from build123d import *

# Parameters (mm, degrees)
SKETCH1_R           = 2.5
SKETCH1_R_2         = 2
BOSS_EXTRUDE1_DEPTH = 0.5
SKETCH3_R           = 2.25
SKETCH3_R_2         = 1.25
BOSS_EXTRUDE2_DEPTH = 6.2
SKETCH5_R           = 3
BOSS_EXTRUDE3_DEPTH = 1.3
SKETCH6_R           = 2.5
BOSS_EXTRUDE4_DEPTH = 6.2
SKETCH24_W          = 5.284246403
SKETCH24_H          = 1
CUT_EXTRUDE1_DEPTH  = 2
FILLET1_R           = 0.5


with BuildPart() as part:
    # Sketch1 → Boss-Extrude1 (new body)
    with BuildSketch(Plane(origin=(0, 0, 0), x_dir=(1, 0, 0), z_dir=(0, 1, 0))):
        with Locations(Location((0, 0, 0), (0, 0, 270))):
            Circle(SKETCH1_R)
        with Locations(Location((0, 0, 0), (0, 0, 270))):
            Circle(SKETCH1_R_2, mode=Mode.SUBTRACT)
    extrude(amount=BOSS_EXTRUDE1_DEPTH)

    # Sketch3 → Boss-Extrude2 (add)
    with BuildSketch(Plane(origin=(0, 0.5, 0), x_dir=(1, 0, 0), z_dir=(0, 1, 0))):
        with Locations(Location((0, 0, 0), (0, 0, 90))):
            Circle(SKETCH3_R)
        with Locations(Location((0, 0, 0), (0, 0, 90))):
            Circle(SKETCH3_R_2, mode=Mode.SUBTRACT)
    extrude(amount=BOSS_EXTRUDE2_DEPTH)

    # Sketch5 → Boss-Extrude3 (add)
    with BuildSketch(Plane(origin=(0, 6.7, 0), x_dir=(1, 0, 0), z_dir=(0, 1, 0))):
        with Locations(Location((0, 0, 0), (0, 0, 270))):
            Circle(SKETCH5_R)
    extrude(amount=BOSS_EXTRUDE3_DEPTH)

    # Sketch6 → Boss-Extrude4 (add)
    with BuildSketch(Plane(origin=(0, 8, 0), x_dir=(1, 0, 0), z_dir=(0, 1, 0))):
        with Locations(Location((0, 0, 0), (0, 0, 270))):
            Circle(SKETCH6_R)
    extrude(amount=BOSS_EXTRUDE4_DEPTH)

    # Sketch24 → Cut-Extrude1 (cut)
    with BuildSketch(Plane(origin=(0, 0, 0), x_dir=(-1, 0, 0), z_dir=(0, -1, 0))):
        with Locations((-0.034581621, 0.031508974)):
            Rectangle(SKETCH24_W, SKETCH24_H)
    extrude(amount=-CUT_EXTRUDE1_DEPTH, mode=Mode.SUBTRACT)

    # Fillet1
    fillet1_edges = [part.edges().sort_by_distance(p)[0] for p in [
        (0, 0.5, 2),
        (0, 0.5, -2),
    ]]
    fillet(fillet1_edges, radius=FILLET1_R - 0.0001)  # a hair under: the kernel refuses the full size


solid = part.part
Check sheet for the modelled part. Datum: model origin and axes. Units: mm. A direction names the side the tool comes from. Round coordinates to 2 decimals unless told otherwise and drop trailing zeros. Order: outer loops, then holes, each group sorted by start corner. A loop starts at its lowest first (then second) coordinate and runs counter-clockwise, first axis right, second up.
Q1. Set-up check for faces 5 (the face through (0.479, 3.557, -1.155)), 6 (the face through (-2.44, 11.06, -0.54)), 7 (the face through (0, 0.2, -2.5)): record each of +Z, -Z, +X, -X, +Y, -Y from which the full face is reachable in a straight line by a thin tool's end or side.
Filled sheet:
face 5: -Y
face 6: +Y
face 7: -Z, -Y
Q2. Cross-section at D-D, the plane y = 11.5. Enter the section's corners in (x, z), plus the area to 3 significant figures.
Filled sheet:
outline: circle Ø5 at (0, 0)
area: 19.6 mm2
Q3. Scan lines: L1, parallel to Z at x = -0.05, y = 3.75; L2, parallel to Y at x = 2.3, z = -1.4. Record each from-to range of solid material in increasing order.
Filled sheet:
L1: z = -2.25 to -1.25, 1.25 to 2.25
L2: y = 6.7 to 8
Q4. Depth check by flat-ended pin: P1, Ø1.4, axis at x = -2, y = 1, coming from the -Z side; P2, Ø1, axis at x = -2, y = 0.5, coming from the +Z side; P3, Ø0.7, axis at x = 1.5, y = 1.5, coming from the +Z side. Enter the tip coordinate at first touch or a pass-through.
Filled sheet:
P1: stops at z = -1.99
P2: stops at z = 2
P3: stops at z = 1.93
Q5. Cross-section at C-C, the plane y = 5. Enter the section's corners in (x, z), plus the area to 3 significant figures.
Filled sheet:
outline: circle Ø4.5 at (0, 0); hole circle Ø2.5 at (0, 0)
area: 11.0 mm2
Q6. Cross-section at A-A, the plane z = 0. Enter the section's corners in (x, y).
Filled sheet:
outline: (-3, 6.7) - (-2.25, 6.7) - (-2.25, 2) - (-1.25, 2) - (-1.25, 6.7) - (1.25, 6.7) - (1.25, 2) - (2.25, 2) - (2.25, 6.7) - (3, 6.7) - (3, 8) - (2.5, 8) - (2.5, 14.2) - (-2.5, 14.2) - (-2.5, 8) - (-3, 8) - close
Q7. Draft check along Z on faces 1 (the face through (2, 1, 0.468)), 2 (the face through (-2, 1, -0.532)), 3 (the face through (2, 8, -2)), 4 (the face through (2.196, 3.557, 0.488)). Enter one of: pulls with the +Z half, pulls with the -Z half, needs draft (parallel to the pull), parting line crosses it, or undercut.
Filled sheet:
face 1: undercut
face 2: undercut
face 3: needs draft
face 4: parting line crosses it
